Work out the finished part from the listing and answer in its coordinate system (mm). Face numbers are marked on the shaded views. A direction names the side the tool comes from. Round coordinates to 2 decimals unless told otherwise and drop trailing zeros. Order: outer loops, then holes, each group sorted by start corner. A loop starts at its lowest first (then second) coordinate and runs counter-clockwise, first axis right, second up. Notation, with made-up numbers: M 11,22 L 28,22 A20 ccw 28,34 Z; hole C 30.5,61.5 d8. An arc over 180 degrees is marked long. Answer as a JSON object with one key per item and string values. Group by question number.
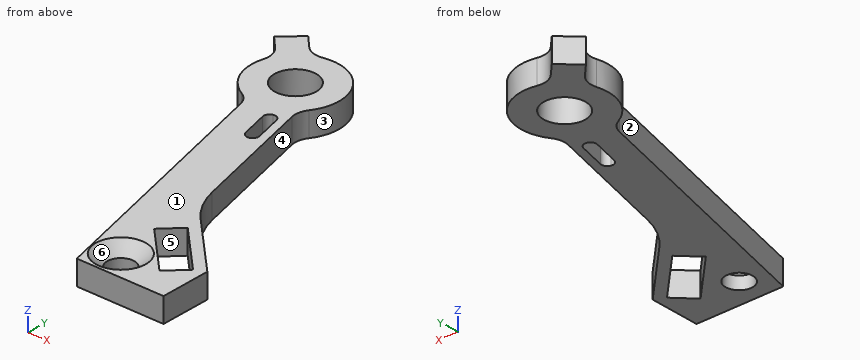
from build123d import *

# Parameters (mm, degrees)
SKETCH1_R           = 1.5
SKETCH1_R_2         = 2.625
BOSS_EXTRUDE1_DEPTH = 3.05
FILLET3_R           = 2.5
FILLET4_R           = 10
FILLET6_R           = 0.75


with BuildPart() as part:
    # Sketch1 → Boss-Extrude1 (new body)
    with BuildSketch(Plane.XY):
        with BuildLine():
            Line((-8.481662584, 34.046021185), (0, 0))
            Line((0, 0), (11, 0))
            Line((11, 0), (11, 6.303908615))
            Line((11, 6.303908615), (1.807611845, 15.496296771))
            Line((1.807611845, 15.496296771), (-3.144779945, 35.375563851))
            ThreePointArc((-3.144779945, 35.375563851), (-2.481245275, 42.518446356), (-9.444822751, 44.241709966))
            Line((-9.444822751, 44.241709966), (-12.046172881, 46.936525265))
            Line((-12.046172881, 46.936525265), (-14.384461968, 44.67933583))
            Line((-14.384461968, 44.67933583), (-11.783111838, 41.984520531))
            ThreePointArc((-11.783111838, 41.984520531), (-12.042982397, 37.220695866), (-8.481662584, 34.046021185))
        make_face()
        with Locations((2.5, 3.5)):
            Circle(SKETCH1_R, mode=Mode.SUBTRACT)
        Polygon((9.727207794, 5.692209589), (7.517499103, 3.482500897), (7.464466094, 3.429467889), (1.701545827, 9.192388155), (3.964287527, 11.455129855), align=None, mode=Mode.SUBTRACT)
        Polygon((-3.942100566, 28.234165792), (-5.150775718, 33.085877281), (-3.695262271, 33.448479827), (-2.48658712, 28.596768337), align=None, mode=Mode.SUBTRACT)
        with Locations((-6.964638989, 39.33266846)):
            Circle(SKETCH1_R_2, mode=Mode.SUBTRACT)
    extrude(amount=BOSS_EXTRUDE1_DEPTH)

    # Sketch3 → CSK for M3 Flat Head Machine Screw1 (revolve, cut)
    with BuildSketch(Plane(origin=(2.5, 3.5, 3.05), x_dir=(0, -1, 0), z_dir=(1, 0, 0))):
        Polygon((0, 0), (0, 3.05), (1.7, 3.05), (1.7, 1.45), (3.15, 0), align=None)
    revolve(axis=Axis((2.5, 3.5, 9.4), (0, 0, -1)), mode=Mode.SUBTRACT)

    # Fillet3
    fillet3_edges = [part.edges().sort_by_distance(p)[0] for p in [
        (-3.144779945, 35.375563851, 1.525),
        (-8.481662584, 34.046021185, 1.525),
        (-11.783111838, 41.984520531, 1.525),
        (-9.444822751, 44.241709966, 1.525),
    ]]
    fillet(fillet3_edges, radius=FILLET3_R)

    # Fillet4
    fillet4_edges = [part.edges().sort_by_distance(p)[0] for p in [
        (1.807611845, 15.496296771, 1.525),
    ]]
    fillet(fillet4_edges, radius=FILLET4_R)

    # Fillet6
    fillet6_edges = [part.edges().sort_by_distance(p)[0] for p in [
        (-2.48658712, 28.596768337, 1.525),
        (-3.942100566, 28.234165792, 1.525),
        (-3.695262271, 33.448479827, 1.525),
        (-5.150775718, 33.085877281, 1.525),
    ]]
    fillet(fillet6_edges, radius=FILLET6_R - 0.0001)  # a hair under: the kernel refuses the full size


solid = part.part
Item 1: Find section C-C (y = 20). Give the vertices of the cut face in (x, z), and give its area (3 significant figures).
Item 2: Consider L1, parallel to Y at x = 2.25, z = 1.75; L2, parallel to X at y = 5, z = 1.9 (3 decimals); L3, parallel to X at y = 8, z = 2.9. Determine where each line is inside the solid, lowest interval first.
Item 3: Each of these flat-tipped pins is pushed along its axis until it touches: pin 1 (4 mm diameter, centred on x = 2.5, y = 3.5, fed in from +Z); pin 2 (1 mm diameter, centred on y = 21, z = 1.5, fed in from +X); pin 3 (1.5 mm diameter, centred on y = 24.5, z = 1, fed in from +X); pin 4 (7 mm diameter, centred on x = -6.96, y = 39.33, fed in from -Z). Where does it stop, or does it pass through?
Item 4: A tool of negligible diameter and unlimited length cuts with its end or side. For the marked faces 4, 5 and 6, from which of +Z, -Z, +X, -X, +Y, -Y can it reach the whole face along a straight path? Write none if from no direction.
Item 5: The mould has two halves that part along Y. Classify the marked faces 1, 2 and 3: +Y half, -Y half, draft (parallel to the pull), parting line (faces both ways), or undercut.
Item 6: Find section B-B (z = 0.55). Give the number of separate pieces and of enclosed holes in the cut face, and give its area (3 significant figures).
Item 7: Find section A-A (x = 2.5). Give the vertices of the cut face in (y, z), and give its area (3 significant figures).
Item 8: Find section D-D (y = 15). Give the vertices of the cut face in (x, z).
Responses:
{
 "1": {"outline": "M -4.98,0 L 0.69,0 L 0.69,3.05 L -4.98,3.05 Z", "area": "17.3 mm^2"},
 "2": {"L1": "y = 0 to 1.67, 5.33 to 8.64, 9.74 to 15.49", "L2": "x = -1.246 to 1.177, 3.823 to 5.894, 9.035 to 11", "L3": "x = -1.99 to 2.89, 7.42 to 9.3"},
 "3": {"pin 1": "stops at z = 1.9", "pin 2": "stops at x = 0.56", "pin 3": "stops at x = -0.25", "pin 4": "stops at z = 0"},
 "4": {"face 4": "+Z, -Z, +X", "face 5": "+Z, -Z", "face 6": "+Z"},
 "5": {"face 1": "draft", "face 2": "-Y half", "face 3": "undercut"},
 "6": {"separate pieces": "1", "enclosed holes": "4", "area": "309 mm^2"},
 "7": {"outline": "M 0,0 L 1.8,0 L 1.8,1.6 L 0.35,3.05 L 0,3.05 Z; M 5.2,0 L 8.39,0 L 8.39,3.05 L 6.65,3.05 L 5.2,1.6 Z; M 9.99,0 L 15.09,0 L 15.09,3.05 L 9.99,3.05 Z", "area": "28.7 mm^2"},
 "8": {"outline": "M -3.74,0 L 2.56,0 L 2.56,3.05 L -3.74,3.05 Z"}
}
